Read the model definition and answer for the solid it produces. Units are mm, in the model's axes. A direction names the side the tool comes from. Give positions to 0.01 mm unless a question says otherwise; leave off trailing zeros. Order: outer loops, then holes, each group sorted by start corner. A loop starts at its lowest first (then second) coordinate and runs counter-clockwise, first axis right, second up. Notation, with made-up numbers: (-26, 47) - (21, 47) arc R9 ccw to (21, 59) - close; hole circle Ø11 at (-2, 30.5). An arc over 180 degrees is marked (long way). Write item = value, one per line.
```python
from build123d import *

# Parameters (mm, degrees)
F0_R     = 20
F1_DEPTH = 30
F2_R     = 30
F3_DEPTH = 40
F4_R     = 60
F5_DEPTH = 180
F6_W     = 60
F6_H     = 110
F7_DEPTH = 39.05434


with BuildPart() as f1:
    # F0 (on Top) → F1 (new body)
    with BuildSketch(Plane.XY):
        Circle(F0_R)
    extrude(amount=-F1_DEPTH)

    # F2 (on Top) → F3 (join)
    with BuildSketch(Plane.XY):
        Circle(F2_R)
    extrude(amount=F3_DEPTH)

    # F4 (on face) → F5 (join)
    with BuildSketch(Plane.XY.offset(40)):
        Circle(F4_R)
    extrude(amount=F5_DEPTH)

    # F6 (on Front) → F7 (cut)
    with BuildSketch(Plane.XZ):
        with Locations((0.414748, 138.215205)):
            Rectangle(F6_W, F6_H)
    extrude(amount=-F7_DEPTH, mode=Mode.SUBTRACT)


solid = f1.part
```
1. Section B-B (z = 176) is taken. Determine the outline of the cut face in (x, y).
Recorded:
outline = circle Ø120 at (0, 0); hole (-29.59, 0) - (30.41, 0) - (30.41, 39.05) - (-29.59, 39.05) - close
2. Straight lines are drawn through the part: L1, parallel to X at y = 1, z = 185; L2, parallel to Z at x = 30, y = -49; L3, parallel to Z at x = 17, y = 38. For each, find the intervals that lie inside material, in ascending order. Write a range as [from, to].
Recorded:
L1 = [-59.99, -29.59], [30.41, 59.99]
L2 = [40, 220]
L3 = [40, 83.22], [193.22, 220]
3. Determine the mould class of faces 4 (the face through (-29.585, 19, 137)), 5 (the face through (0, 0, 139)), 6 (the face through (-29.97, 1.32, 19.72)), 7 (the face through (12, 28, 40)) for opening direction X: +X half, -X half, draft (parallel to the pull), parting line (faces both ways), or undercut.
Recorded:
face_4 = undercut
face_5 = undercut
face_6 = parting line
face_7 = draft
4. Section D-D (y = 6) is taken. Determine the outline of the cut face in (x, z).
Recorded:
outline = (-59.7, 40) - (-29.39, 40) - (-29.39, 0) - (-19.08, 0) - (-19.08, -30) - (19.08, -30) - (19.08, 0) - (29.39, 0) - (29.39, 40) - (59.7, 40) - (59.7, 220) - (-59.7, 220) - close; hole (-29.59, 83.22) - (30.41, 83.22) - (30.41, 193.22) - (-29.59, 193.22) - close
5. Flat-ended cylindrical pins translate along their axes: pin 1 (5 mm diameter, centred on x = -29, y = -6, fed in from -Z); pin 2 (3 mm diameter, centred on y = 17, z = 115, fed in from -X); pin 3 (4 mm diameter, centred on x = -10, y = 34.5, fed in from -Z). Find the tip coordinate at first contact, or state that the pin passes through.
Recorded:
pin_1 = 0
pin_2 = -57.96
pin_3 = 40
6. For faces 1 (the face through (6, -20, 0)), 2 (the face through (0, 19, 83.215)), 3 (the face through (0, 0, -30)), determine the directions among +Z, -Z, +X, -X, +Y, -Y from which every point of the face is accessible in a straight line to the end or side of a thin tool.
Recorded:
face_1 = -Z
face_2 = none
face_3 = -Z, +X, -X, +Y, -Y
7. Section A-A (x = 0) is taken. Determine the outline of the cut face in (y, z), and give its area (3 significant figures).
Recorded:
outline = (-60, 40) - (-30, 40) - (-30, 0) - (-20, 0) - (-20, -30) - (20, -30) - (20, 0) - (30, 0) - (30, 40) - (60, 40) - (60, 220) - (-60, 220) - close; hole (0, 83.22) - (39.05, 83.22) - (39.05, 193.22) - (0, 193.22) - close
area = 20,900 mm^2
8. Section C-C (y = -24.5) is taken. Determine the outline of the cut face in (x, z).
Recorded:
outline = (-54.77, 40) - (-17.31, 40) - (-17.31, 0) - (17.31, 0) - (17.31, 40) - (54.77, 40) - (54.77, 220) - (-54.77, 220) - close
